Autodesk Inventor part; units mm, degrees
ref_plane "YZ Plane" through (0, 0, 0) normal (1, 0, 0) x (0, 1, 0)
ref_plane "XZ Plane" through (0, 0, 0) normal (0, 1, 0) x (-1, 0, 0)
ref_plane "XY Plane" through (0, 0, 0) normal (0, 0, 1) x (1, 0, 0)
sketch "Sketch1" plane through (0, 0, 0) normal (0, 1, 0) x (-1, 0, 0)
  line L0 (40, 29) -> (-40, 29)
  line L1 (-40, 29) -> (-40, 11)
  line L2 (-40, 11) -> (40, 11)
  line L3 (40, 11) -> (40, 29)
  line L4 (40, -11) -> (-40, -11)
  line L5 (-40, -11) -> (-40, -29)
  line L6 (-40, -29) -> (40, -29)
  line L7 (40, -29) -> (40, -11)
  line L8 (40, 11) -> (40, -11) construction
  point P0 (0, 0)
  point P1 (40, 0)
  point P2 (0, 29)
  dimension "d0" = 58
  dimension "d1" = 18
  dimension "d2" = 80
extrude "Extrusion1" add sketch "Sketch1" along normal blind 4
sketch "Sketch2" plane through (0, 4, 0) normal (0, 1, 0) x (1, 0, 0)
  line L0 (40, -29) -> (40, -11)
  line L1 (-40, -11) -> (40, -11)
  line L2 (40, -11) -> (40, -14)
  line L3 (40, -14) -> (-40, -14)
  line L4 (-40, -14) -> (-40, -11)
  line L5 (40, 11) -> (40, 29)
  line L6 (-40, 11) -> (40, 11)
  line L7 (40, 11) -> (40, 14)
  line L8 (40, 14) -> (-40, 14)
  line L9 (-40, 14) -> (-40, 11)
  point P0 (0, 0)
  dimension "d5" = 3
  dimension "d6" = 3
extrude "Extrusion2" add sketch "Sketch2" along normal blind 4
sketch "Sketch3" plane through (0, 8, 0) normal (0, 1, 0) x (1, 0, 0)
  line L0 (-40, -14) -> (40, -14)
  line L1 (40, 11) -> (40, 29)
  line L2 (-40, -14) -> (40, -14)
  line L3 (40, -14) -> (40, 14)
  line L4 (40, 14) -> (-40, 14)
  line L5 (-40, 14) -> (-40, -14)
  point P0 (0, 0)
extrude "Extrusion3" add sketch "Sketch3" along normal blind 3
sketch "Sketch4" plane through (0, 4, 0) normal (0, 1, 0) x (1, 0, 0)
  line L0 (-40, -29) -> (40, -29)
  line L1 (40, 29) -> (-40, 29)
  line L2 (-40, 29) -> (-40, 14)
  line L3 (40, 14) -> (40, 29)
  point P0 (0, 0)
  point P1 (-20, -20)
  point P2 (20, -20)
  point P3 (-20, 20)
  point P4 (20, 20)
  dimension "d12" = 9
  dimension "d13" = 9
  dimension "d14" = 20
  dimension "d15" = 20
hole "Hole1" at (-20, 4, 20) at (20, 4, 20) at (-20, 4, -20) at (20, 4, -20) direction (0, -1, 0) diameter 5.5 end through all
properties part number "Main Carriage - Wheel Base"
Here's how the part is built. I have some questions about the finished solid (model axes, mm). A direction names the side the tool comes from. Give positions to 0.01 mm unless a question says otherwise; leave off trailing zeros. Loops run counter-clockwise (first coordinate to the right, second up) from the corner with the lowest first, then second, coordinate; pieces in that order, holes last. Notation, with made-up numbers: (-11, 86) -> (23, 86) arc R23 ccw to (23, 118) -> close; hole circle Ø8 at (28.25, 86.25). An arc over 180 degrees is marked (long way). Use one line per item in the form item = value. Start each with the question number.
1) Please list where these lines run through material, in increasing order: line 1 along X through (y, z) = (2.05, 20); line 2 along Z through (x, y) = (-20, 1.05); line 3 along Z through (x, y) = (32, 3.5).
2) Which directions (+Z, -Z, +X, -X, +Y, -Y) give clear straight access to the entire face, cutting with the end or side of a thin tool? Please do faces 4 (the face through (-1, 11, 0)), 5 (the face through (19.879, 1.972, -22.747)), 6 (the face through (-1, 8, 0)), 7 (the face through (1, 7, -14)), 8 (the face through (-1, 7, 14)).
3) Thinking about a two-plate mould opening in Z: for faces 1 (the face through (1, 4, 22)), 2 (the face through (19.879, 1.972, 17.253)), 3 (the face through (1, 2, -29)), which applies, +Z half, -Z half, draft (parallel to the pull), parting line (faces both ways), or undercut?
4) Imagine slicing it at C-C (z = 20). Please give me the cut outline in (x, y).
5) Imagine slicing it at D-D (y = 1). Please give me the cut outline in (x, z).
6) Imagine slicing it at A-A (x = 20). Please give me the cut outline in (y, z), then the cut area to 3 significant figures.
7) Imagine slicing it at B-B (y = 6.25). Please give me the cut outline in (x, z), then the cut area to 3 significant figures.
8) For P1, Ø5, axis at x = -7.5, z = -22, coming from the +Y side; P2, Ø5.5, axis at x = -10, y = 7, coming from the -Z side; P3, Ø5, axis at x = -4, y = 8.5, coming from the +Z side, each with a flat end and sliding along its axis, tell me the tip position at first contact or that it passes through.
Check values:
q1.line_1 = -40 to -22.75, -17.25 to 17.25, 22.75 to 40
q1.line_2 = -29 to -22.75, -17.25 to -11, 11 to 17.25, 22.75 to 29
q1.line_3 = -29 to -11, 11 to 29
q2.face_4 = +Z, -Z, +X, -X, +Y
q2.face_5 = +Y, -Y
q2.face_6 = +X, -X, -Y
q2.face_7 = -Z, +X, -X, +Y
q2.face_8 = +Z, +X, -X, +Y
q3.face_1 = draft
q3.face_2 = undercut
q3.face_3 = -Z half
q4.outline = (-40, 0) -> (-22.75, 0) -> (-22.75, 4) -> (-40, 4) -> close; (-17.25, 0) -> (17.25, 0) -> (17.25, 4) -> (-17.25, 4) -> close; (22.75, 0) -> (40, 0) -> (40, 4) -> (22.75, 4) -> close
q5.outline = (-40, -29) -> (40, -29) -> (40, -11) -> (-40, -11) -> close; (-40, 11) -> (40, 11) -> (40, 29) -> (-40, 29) -> close; hole circle Ø5.5 at (-20, -20); hole circle Ø5.5 at (-20, 20); hole circle Ø5.5 at (20, -20); hole circle Ø5.5 at (20, 20)
q6.outline = (0, -29) -> (4, -29) -> (4, -22.75) -> (0, -22.75) -> close; (0, -17.25) -> (4, -17.25) -> (4, -14) -> (11, -14) -> (11, 14) -> (4, 14) -> (4, 17.25) -> (0, 17.25) -> (0, 11) -> (8, 11) -> (8, -11) -> (0, -11) -> close; (0, 22.75) -> (4, 22.75) -> (4, 29) -> (0, 29) -> close
q6.area = 208 mm^2
q7.outline = (-40, -14) -> (40, -14) -> (40, -11) -> (-40, -11) -> close; (-40, 11) -> (40, 11) -> (40, 14) -> (-40, 14) -> close
q7.area = 480 mm^2
q8.P1 = 4
q8.P2 = -14
q8.P3 = 14
